Check sheet for the modelled part. Datum: model origin and axes. Units: mm. A direction names the side the tool comes from. Coordinates: 2 decimals unless noted, no trailing zeros. Order: outer loops, then holes, each group sorted by start corner. A loop starts at its lowest first (then second) coordinate and runs counter-clockwise, first axis right, second up.
Autodesk Inventor part; units mm, degrees
ref_plane "YZ Plane" through (0, 0, 0) normal (1, 0, 0) x (0, 1, 0)
ref_plane "XZ Plane" through (0, 0, 0) normal (0, 1, 0) x (-1, 0, 0)
ref_plane "XY Plane" through (0, 0, 0) normal (0, 0, 1) x (1, 0, 0)
sketch "Sketch1" plane through (0, 0, 0) normal (0, 0, 1) x (1, 0, 0)
  line L0 (8.65, 3.5829) -> (8.65, -3.5829)
  line L1 (8.65, -3.5829) -> (3.5829, -8.65)
  line L2 (3.5829, -8.65) -> (-3.5829, -8.65)
  line L3 (-3.5829, -8.65) -> (-8.65, -3.5829)
  line L4 (-8.65, -3.5829) -> (-8.65, 3.5829)
  line L5 (-8.65, 3.5829) -> (-3.5829, 8.65)
  line L6 (-3.5829, 8.65) -> (3.5829, 8.65)
  line L7 (3.5829, 8.65) -> (8.65, 3.5829)
  line L8 (-12.7904, 0) -> (12.7904, 0)
  line L9 (12.7904, 0) -> (12.7904, -18.65)
  line L10 (12.7904, -18.65) -> (-12.7904, -18.65)
  line L11 (-12.7904, -18.65) -> (-12.7904, 0)
  point P0 (0, 0)
  point P1 (0, 0)
  point P2 (0, 0)
  point P3 (-8.65, 0)
  point P4 (8.65, 0)
  dimension "d0" = 17.3
  dimension "d1" = 10
extrude "Extrusion1" add sketch "Sketch1" along normal blind 18 contours L8 L9 L10 L11 L4 L3 L2 L1 L0
sketch "Sketch2" plane through (0, 0, 0) normal (0, 0, -1) x (-1, 0, 0)
  line L0 (-12.7904, -18.65) -> (-12.7904, 0)
  line L1 (12.7904, 0) -> (12.7904, -18.65)
  line L2 (-12.7904, -18.65) -> (12.7904, -18.65)
  line L3 (12.7904, -18.65) -> (12.7904, -9.275)
  line L4 (12.7904, -9.325) -> (-12.7904, -9.325)
  line L5 (-12.7904, -9.325) -> (-12.7904, -18.65)
  point P0 (0, 0)
  point P1 (-12.7904, -9.325)
extrude "Extrusion2" add sketch "Sketch2" along normal blind 31
extrude "Extrusion3" add sketch "Sketch1" against normal blind 18 from surface at -31 contours L8 L9 L10 L11 L4 L3 L2 L1 L0
sketch "Sketch3" plane through (12.7904, -18.65, 18) normal (1, 0, 0) x (0, 0, -1)
  line L0 (29.5, 6.5107) -> (37.5, 6.5107)
  line L1 (37.5, 6.5107) -> (37.5, 3.0107)
  line L2 (37.5, 3.0107) -> (29.5, 3.0107)
  line L3 (29.5, 3.0107) -> (29.5, 6.5107)
  line L4 (29.5, 6.5107) -> (37.5, 3.0107) construction
  line L5 (37.5, 6.5107) -> (29.5, 3.0107) construction
  line L6 (18, 9.325) -> (49, 9.325)
  point P0 (18, 18.65)
  point P1 (33.5, 4.7607)
  point P2 (33.5, 9.325)
  dimension "d8" = 3.5
  dimension "d9" = 8
extrude "Extrusion4" cut sketch "Sketch3" against normal through all
properties part number "Gage Stand"
(1) Cross-section at D-D (y = -2.75). Enter the section's corners in (x, z).
Filled in:
outline: (-12.79, -49) - (-8.65, -49) - (-8.65, -31) - (-12.79, -31) - close; (-12.79, 0) - (-8.65, 0) - (-8.65, 18) - (-12.79, 18) - close; (8.65, -49) - (12.79, -49) - (12.79, -31) - (8.65, -31) - close; (8.65, 0) - (12.79, 0) - (12.79, 18) - (8.65, 18) - close
(2) Tool access check on faces 1 (the flat face through (0, -12.139, -15)), 2 (the flat face through (0, -9, -31)), 3 (the flat face through (6.152, -6.081, 8.874)), 4 (the flat face through (12.79, -11, -15)), 5 (the flat face through (0, -18.65, -15)). Record the directions out of +Z, -Z, +X, -X, +Y, -Y that give a thin tool (end or side, any length) a straight path to the whole face; none if there is none.
Filled in:
face 1: +X, -X
face 2: +X, -X, +Y
face 3: +Z, -Z, +Y
face 4: +Z, -Z, +X, +Y, -Y
face 5: +Z, -Z, +X, -X, -Y
(3) Release check for a two-part mould opening along Z. For faces 6 (the flat face through (0, -11, 18)), 7 (the flat face through (0, -14, -11.5)), 8 (the flat face through (-6.081, -6.152, 8.874)) record: +Z half, -Z half, draft (parallel to the pull), parting line (faces both ways), or undercut.
Filled in:
face 6: +Z half
face 7: undercut
face 8: draft
(4) Go/stop test with flat-tipped pins: P1, Ø5, axis at x = -6.5, z = -9, coming from the +Y side (3 decimals); P2, Ø8, axis at x = 0, z = 9.5, coming from the +Y side. Record where each tip stops, or that it passes through.
Filled in:
P1: stops at y = -9.325
P2: stops at y = -8.23
(5) Cross-section at B-B (z = -16.5). Enter the section's corners in (x, y) (3 decimals), and give its area (3 significant figures).
Filled in:
outline: (-12.79, -18.65) - (12.79, -18.65) - (12.79, -15.639) - (-12.79, -15.639) - close; (-12.79, -12.139) - (12.79, -12.139) - (12.79, -9.325) - (-12.79, -9.325) - close
area: 149 mm2
(6) Cross-section at C-C (x = -2.25). Enter the section's corners in (y, z) (3 decimals).
Filled in:
outline: (-18.65, -49) - (-8.65, -49) - (-8.65, -31) - (-9.325, -31) - (-9.325, 0) - (-8.65, 0) - (-8.65, 18) - (-18.65, 18) - close; hole (-15.639, -19.5) - (-12.139, -19.5) - (-12.139, -11.5) - (-15.639, -11.5) - close
(7) Thickness scan on probe 1 along Z at (x, y) = (9.75, -6.25); probe 2 along Z at (x, y) = (7, -14.5); probe 3 along X at (y, z) = (-1, -35). Record the ranges inside material, lowest first.
Filled in:
probe 1: z = -49 to -31, 0 to 18
probe 2: z = -49 to -19.5, -11.5 to 18
probe 3: x = -12.79 to -8.65, 8.65 to 12.79
(8) Cross-section at A-A (y = -14.25). Enter the section's corners in (x, z), and give its area (3 significant figures).
Filled in:
outline: (-12.79, -49) - (12.79, -49) - (12.79, -19.5) - (-12.79, -19.5) - close; (-12.79, -11.5) - (12.79, -11.5) - (12.79, 18) - (-12.79, 18) - close
area: 1,510 mm2
